```python
from build123d import *

# Parameters (mm, degrees)
SKETCH_1_W          = 14
SKETCH_1_H          = 14
SKETCH_1_W_2        = 10
SKETCH_1_H_2        = 10
EXTRUDE_1_DEPTH     = 10
SKETCH_2_W          = 14
SKETCH_2_H          = 14
EXTRUDE_2_DEPTH     = 5
SKETCH_3_W          = 14
SKETCH_3_H          = 14
SKETCH_3_W_2        = 10
SKETCH_3_H_2        = 10
EXTRUDE_3_DEPTH     = 10
SKETCH_6_R          = 1
CUT_EXTRUDE_1_DEPTH = 16


with BuildPart() as part:
    # 草图1 → 凸台-拉伸1 (new body)
    with BuildSketch(Plane.XY):
        with Locations((7, 7)):
            Rectangle(SKETCH_1_W, SKETCH_1_H)
        with Locations((7, 7)):
            Rectangle(SKETCH_1_W_2, SKETCH_1_H_2, mode=Mode.SUBTRACT)
    extrude(amount=EXTRUDE_1_DEPTH)

    # 草图2 → 凸台-拉伸2 (add)
    with BuildSketch(Plane.XY.offset(10)):
        with Locations((7, 7)):
            Rectangle(SKETCH_2_W, SKETCH_2_H)
    extrude(amount=EXTRUDE_2_DEPTH)

    # 草图3 → 凸台-拉伸3 (add)
    with BuildSketch(Plane.XY.offset(15)):
        with Locations((7, 7)):
            Rectangle(SKETCH_3_W, SKETCH_3_H)
        with Locations((7, 7)):
            Rectangle(SKETCH_3_W_2, SKETCH_3_H_2, mode=Mode.SUBTRACT)
    extrude(amount=EXTRUDE_3_DEPTH)

    # 草图6 → 切除-拉伸1 (cut)
    with BuildSketch(Plane(origin=(14, 0, 0), x_dir=(0, 0, -1), z_dir=(1, 0, 0))):
        with Locations((-12.5, 8)):
            Circle(SKETCH_6_R)
    extrude(amount=-CUT_EXTRUDE_1_DEPTH, mode=Mode.SUBTRACT)


solid = part.part
```
For this review, take the finished solid that the model builds, in its own axes (mm). A direction names the side the tool comes from. Round coordinates to 2 decimals unless told otherwise and drop trailing zeros. Loops run counter-clockwise (first coordinate to the right, second up) from the corner with the lowest first, then second, coordinate; pieces in that order, holes last.
Q1. Insertion check: pin 1 Ø8 at (x, y) = (7, 6.5) entering from +Z. The pin has a flat end and moves straight along its axis. Give the tip position at first contact, or say it passes through.
Result sheet:
pin 1: stops at z = 15
Q2. Add section B-B on z = 12.5. Write out the cut boundary in (x, y).
Result sheet:
outline: (0, 0) - (14, 0) - (14, 7) - (0, 7) - close; (0, 9) - (14, 9) - (14, 14) - (0, 14) - close
Q3. Add section C-C on x = 3.25. Write out the cut boundary in (y, z).
Result sheet:
outline: (0, 0) - (2, 0) - (2, 10) - (12, 10) - (12, 0) - (14, 0) - (14, 25) - (12, 25) - (12, 15) - (2, 15) - (2, 25) - (0, 25) - close; hole circle Ø2 at (8, 12.5)
Q4. Machinability: for faces 1 (the face through (12, 7, 20)), 2 (the face through (2, 7, 5)), 3 (the face through (1, 7, 0)), which of the approach directions +Z, -Z, +X, -X, +Y, -Y give a long, thin tool a straight path to every point of the face, cutting with its end or side? Answer none if there is none.
Result sheet:
face 1: +Z
face 2: -Z
face 3: -Z, +X, -X, +Y, -Y
Q5. Mouldability with a two-part tool opening along X and no side actions: class faces 4 (the face through (7, 2, 5)), 5 (the face through (1, 7, 25)), 6 (the face through (14, 5, 12)) as +X half, -X half, draft (parallel to the pull), parting line (faces both ways), or undercut.
Result sheet:
face 4: undercut
face 5: draft
face 6: +X half
Q6. Add section A-A on y = 8. Write out the cut boundary in (x, z), plus the area to 3 significant figures.
Result sheet:
outline: (0, 0) - (2, 0) - (2, 10) - (12, 10) - (12, 0) - (14, 0) - (14, 11.5) - (0, 11.5) - close; (0, 13.5) - (14, 13.5) - (14, 25) - (12, 25) - (12, 15) - (2, 15) - (2, 25) - (0, 25) - close
area: 122 mm2
Q7. Add section D-D on z = 18. Write out the cut boundary in (x, y).
Result sheet:
outline: (0, 0) - (14, 0) - (14, 14) - (0, 14) - close; hole (2, 2) - (12, 2) - (12, 12) - (2, 12) - close
Q8. To check wall thickness, follow line 1 along X through (y, z) = (8.25, 4.25); line 2 along Y through (x, z) = (10.75, 12.5); line 3 along Z through (x, y) = (11.5, 11.25). State the ranges of each line that lie inside material, in increasing order.
Result sheet:
line 1: x = 0 to 2, 12 to 14
line 2: y = 0 to 7, 9 to 14
line 3: z = 10 to 15
